```python
from build123d import *

# Parameters (mm, degrees)
SKETCH_1_W               = 50
SKETCH_1_H               = 50
EXTRUDE_1_DEPTH          = 5
CUT_EXTRUDE_1_REACH      = 37.707
SKETCH_2_R               = 15
SKETCH_3_R               = 22.5
CUT_EXTRUDE_2_DEPTH      = 3
CUT_EXTRUDE_3_REACH      = 37.482
SKETCH_4_R               = 1.25
CHAMFER_1_SIZE           = 1
EXTRUDE_2_DEPTH          = 1.5
EXTRUDE_START            = 20
EXTRUDE_3_DEPTH          = 20
CUT_EXTRUDE_4_REACH      = 59.228
SKETCH_9_R               = 1.65
CUT_EXTRUDE_5_DEPTH      = 3
MIRROR_1_COPY_1_REACH    = 59.228
MIRROR_1_COPY_1_SKETCH_R = 1.65
MIRROR_1_COPY_2_DEPTH    = 3


with BuildPart() as part:
    # Sketch 1 → Extrude 1 (new body)
    with BuildSketch(Plane(origin=(0, 0, 0), x_dir=(1, 0, 0), z_dir=(0, 1, 0))):
        Rectangle(SKETCH_1_W, SKETCH_1_H)
    extrude(amount=EXTRUDE_1_DEPTH)

    # Sketch 2 → Cut-Extrude 1 (cut, up to next)
    with BuildSketch(Plane(origin=(0, 5, 0), x_dir=(1, 0, 0), z_dir=(0, 1, 0)), mode=Mode.PRIVATE) as cut_extrude_1_sk1:
        with Locations(Location((0, 0, 0), (0, 0, 270))):
            Circle(SKETCH_2_R)
    cut_extrude_1_tool1 = extrude(cut_extrude_1_sk1.sketch, amount=-CUT_EXTRUDE_1_REACH, mode=Mode.PRIVATE) & part.part
    add(cut_extrude_1_tool1.solids().sort_by_distance((0, 5, 0))[0], mode=Mode.SUBTRACT)

    # Sketch 3 → Cut-Extrude 2 (cut)
    with BuildSketch(Plane(origin=(0, 5, 0), x_dir=(1, 0, 0), z_dir=(0, 1, 0))):
        with Locations(Location((0, 0, 0), (0, 0, 270))):
            Circle(SKETCH_3_R)
    extrude(amount=-CUT_EXTRUDE_2_DEPTH, mode=Mode.SUBTRACT)

    # Sketch 4 → Cut-Extrude 3 (cut, up to next)
    with BuildSketch(Plane(origin=(0, 2, 0), x_dir=(1, 0, 0), z_dir=(0, 1, 0)), mode=Mode.PRIVATE) as cut_extrude_3_sk1:
        with Locations(Location((0, -18.5, 0), (0, 0, 270))):
            Circle(SKETCH_4_R)
    cut_extrude_3_tool1 = extrude(cut_extrude_3_sk1.sketch, amount=-CUT_EXTRUDE_3_REACH, mode=Mode.PRIVATE) & part.part
    # Sketch 4 → Cut-Extrude 3 (cut, up to next)
    with BuildSketch(Plane(origin=(0, 2, 0), x_dir=(1, 0, 0), z_dir=(0, 1, 0)), mode=Mode.PRIVATE) as cut_extrude_3_sk2:
        with Locations(Location((-16.02146997, 9.25, 0), (0, 0, 270))):
            Circle(SKETCH_4_R)
    cut_extrude_3_tool2 = extrude(cut_extrude_3_sk2.sketch, amount=-CUT_EXTRUDE_3_REACH, mode=Mode.PRIVATE) & part.part
    # Sketch 4 → Cut-Extrude 3 (cut, up to next)
    with BuildSketch(Plane(origin=(0, 2, 0), x_dir=(1, 0, 0), z_dir=(0, 1, 0)), mode=Mode.PRIVATE) as cut_extrude_3_sk3:
        with Locations(Location((16.02146997, 9.25, 0), (0, 0, 270))):
            Circle(SKETCH_4_R)
    cut_extrude_3_tool3 = extrude(cut_extrude_3_sk3.sketch, amount=-CUT_EXTRUDE_3_REACH, mode=Mode.PRIVATE) & part.part
    add(cut_extrude_3_tool1.solids().sort_by_distance((0, 2, 18.5))[0], mode=Mode.SUBTRACT)
    add(cut_extrude_3_tool2.solids().sort_by_distance((-16.02147, 2, -9.25))[0], mode=Mode.SUBTRACT)
    add(cut_extrude_3_tool3.solids().sort_by_distance((16.02147, 2, -9.25))[0], mode=Mode.SUBTRACT)

    # Chamfer 1
    chamfer_1_edges = [part.edges().sort_by_distance(p)[0] for p in [
        (0, 2, -22.5),
    ]]
    chamfer(chamfer_1_edges, length=CHAMFER_1_SIZE)

    # Sketch 7 → Extrude 2 (add)
    with BuildSketch(Plane(origin=(0, 2, 0), x_dir=(1, 0, 0), z_dir=(0, 1, 0))):
        with BuildLine():
            ThreePointArc((-5.137558045, 19.173627652), (-9.925, 17.190604265), (-14.036069607, 14.036069607))
            ThreePointArc((-14.036069607, 14.036069607), (-14.036069607, 11.773327907), (-11.773327907, 11.773327907))
            ThreePointArc((-11.773327907, 11.773327907), (-8.325, 14.419322973), (-4.309337101, 16.082665008))
            ThreePointArc((-4.309337101, 16.082665008), (-3.177966251, 18.042256802), (-5.137558045, 19.173627652))
        make_face()
        with BuildLine():
            ThreePointArc((14.036069607, 14.036069607), (9.925, 17.190604265), (5.137558045, 19.173627652))
            ThreePointArc((5.137558045, 19.173627652), (3.177966251, 18.042256802), (4.309337101, 16.082665008))
            ThreePointArc((4.309337101, 16.082665008), (8.325, 14.419322973), (11.773327907, 11.773327907))
            ThreePointArc((11.773327907, 11.773327907), (14.036069607, 11.773327907), (14.036069607, 14.036069607))
        make_face()
        with BuildLine():
            ThreePointArc((19.173627652, -5.137558045), (19.85, 0), (19.173627652, 5.137558045))
            ThreePointArc((19.173627652, 5.137558045), (17.214035858, 6.268928895), (16.082665008, 4.309337101))
            ThreePointArc((16.082665008, 4.309337101), (16.65, 0), (16.082665008, -4.309337101))
            ThreePointArc((16.082665008, -4.309337101), (17.214035858, -6.268928895), (19.173627652, -5.137558045))
        make_face()
        with BuildLine():
            ThreePointArc((5.137558045, -19.173627652), (9.925, -17.190604265), (14.036069607, -14.036069607))
            ThreePointArc((14.036069607, -14.036069607), (14.036069607, -11.773327907), (11.773327907, -11.773327907))
            ThreePointArc((11.773327907, -11.773327907), (8.325, -14.419322973), (4.309337101, -16.082665008))
            ThreePointArc((4.309337101, -16.082665008), (3.177966251, -18.042256802), (5.137558045, -19.173627652))
        make_face()
        with BuildLine():
            ThreePointArc((-14.036069607, -14.036069607), (-9.925, -17.190604265), (-5.137558045, -19.173627652))
            ThreePointArc((-5.137558045, -19.173627652), (-3.177966251, -18.042256802), (-4.309337101, -16.082665008))
            ThreePointArc((-4.309337101, -16.082665008), (-8.325, -14.419322973), (-11.773327907, -11.773327907))
            ThreePointArc((-11.773327907, -11.773327907), (-14.036069607, -11.773327907), (-14.036069607, -14.036069607))
        make_face()
        with BuildLine():
            ThreePointArc((-19.173627652, 5.137558045), (-19.85, 0), (-19.173627652, -5.137558045))
            ThreePointArc((-19.173627652, -5.137558045), (-17.214035858, -6.268928895), (-16.082665008, -4.309337101))
            ThreePointArc((-16.082665008, -4.309337101), (-16.65, 0), (-16.082665008, 4.309337101))
            ThreePointArc((-16.082665008, 4.309337101), (-17.214035858, 6.268928895), (-19.173627652, 5.137558045))
        make_face()
    extrude(amount=EXTRUDE_2_DEPTH)

    # Sketch 8 → Extrude 3 (add)
    with BuildSketch(Plane(origin=(0, 5, 0), x_dir=(1, 0, 0), z_dir=(0, 1, 0)).offset(EXTRUDE_START)):
        with BuildLine():
            Line((-25, -25), (25, -25))
            Line((25, -25), (25, -20))
            Line((25, -20), (10.307764064, -20))
            ThreePointArc((10.307764064, -20), (0, -22.5), (-10.307764064, -20))
            Line((-10.307764064, -20), (-25, -20))
            Line((-25, -20), (-25, -25))
        make_face()
    extrude_3 = extrude(amount=-EXTRUDE_3_DEPTH)

    # Sketch 9 → Cut-Extrude 4 (cut, up to next)
    with BuildSketch(Plane(origin=(0, 0, 20), x_dir=(-1, 0, 0), z_dir=(0, 0, -1)), mode=Mode.PRIVATE) as cut_extrude_4_sk1:
        with Locations((21, 21)):
            Circle(SKETCH_9_R)
    cut_extrude_4_tool1 = extrude(cut_extrude_4_sk1.sketch, amount=-CUT_EXTRUDE_4_REACH, mode=Mode.PRIVATE) & part.part
    # Sketch 9 → Cut-Extrude 4 (cut, up to next)
    with BuildSketch(Plane(origin=(0, 0, 20), x_dir=(-1, 0, 0), z_dir=(0, 0, -1)), mode=Mode.PRIVATE) as cut_extrude_4_sk2:
        with Locations((21, 9)):
            Circle(SKETCH_9_R)
    cut_extrude_4_tool2 = extrude(cut_extrude_4_sk2.sketch, amount=-CUT_EXTRUDE_4_REACH, mode=Mode.PRIVATE) & part.part
    cut_extrude_4_1 = cut_extrude_4_tool1.solids().sort_by_distance((-21, 21, 20))[0]
    add(cut_extrude_4_1, mode=Mode.SUBTRACT)
    cut_extrude_4_2 = cut_extrude_4_tool2.solids().sort_by_distance((-21, 9, 20))[0]
    add(cut_extrude_4_2, mode=Mode.SUBTRACT)
    cut_extrude_4 = cut_extrude_4_1 + cut_extrude_4_2  # Cut-Extrude 4 as one shape, for the pattern or mirror that repeats it

    # Sketch 10 → Cut-Extrude 5 (cut)
    with BuildSketch(Plane(origin=(0, 0, 20), x_dir=(-1, 0, 0), z_dir=(0, 0, -1))):
        Polygon((24.290896534, 21), (22.645448267, 23.85), (19.354551733, 23.85), (17.709103466, 21), (19.354551733, 18.15), (22.645448267, 18.15), align=None)
        Polygon((24.290896534, 9), (22.645448267, 11.85), (19.354551733, 11.85), (17.709103466, 9), (19.354551733, 6.15), (22.645448267, 6.15), align=None)
    cut_extrude_5 = extrude(amount=-CUT_EXTRUDE_5_DEPTH, mode=Mode.SUBTRACT)

    # Mirror 2: Cut-Extrude 4, Cut-Extrude 5 across plane
    add(cut_extrude_4.mirror(Plane(origin=(0, 0, 0), x_dir=(0, 0, 1), z_dir=(1, 0, 0))), mode=Mode.SUBTRACT)
    add(cut_extrude_5.mirror(Plane(origin=(0, 0, 0), x_dir=(0, 0, 1), z_dir=(1, 0, 0))), mode=Mode.SUBTRACT)

    # Mirror 1: Extrude 3, Cut-Extrude 4, Cut-Extrude 5 across plane
    add(extrude_3.mirror(Plane.XY))
    add(cut_extrude_4.mirror(Plane.XY), mode=Mode.SUBTRACT)
    add(cut_extrude_5.mirror(Plane.XY), mode=Mode.SUBTRACT)

    # Mirror 1 copy 1 sketch → Mirror 1 copy 1 (cut, up to next)
    with BuildSketch(Plane.XY.offset(-20), mode=Mode.PRIVATE) as mirror_1_copy_1_sk1:
        with Locations((21, 21)):
            Circle(MIRROR_1_COPY_1_SKETCH_R)
    mirror_1_copy_1_tool1 = extrude(mirror_1_copy_1_sk1.sketch, amount=-MIRROR_1_COPY_1_REACH, mode=Mode.PRIVATE) & part.part
    # Mirror 1 copy 1 sketch → Mirror 1 copy 1 (cut, up to next)
    with BuildSketch(Plane.XY.offset(-20), mode=Mode.PRIVATE) as mirror_1_copy_1_sk2:
        with Locations((21, 9)):
            Circle(MIRROR_1_COPY_1_SKETCH_R)
    mirror_1_copy_1_tool2 = extrude(mirror_1_copy_1_sk2.sketch, amount=-MIRROR_1_COPY_1_REACH, mode=Mode.PRIVATE) & part.part
    add(mirror_1_copy_1_tool1.solids().sort_by_distance((21, 21, -20))[0], mode=Mode.SUBTRACT)
    add(mirror_1_copy_1_tool2.solids().sort_by_distance((21, 9, -20))[0], mode=Mode.SUBTRACT)

    # Mirror 1 copy 2 sketch → Mirror 1 copy 2 (cut)
    with BuildSketch(Plane.XY.offset(-20)):
        Polygon((24.290896534, 21), (22.645448267, 23.85), (19.354551733, 23.85), (17.709103466, 21), (19.354551733, 18.15), (22.645448267, 18.15), align=None)
        Polygon((24.290896534, 9), (22.645448267, 11.85), (19.354551733, 11.85), (17.709103466, 9), (19.354551733, 6.15), (22.645448267, 6.15), align=None)
    extrude(amount=-MIRROR_1_COPY_2_DEPTH, mode=Mode.SUBTRACT)


solid = part.part
```
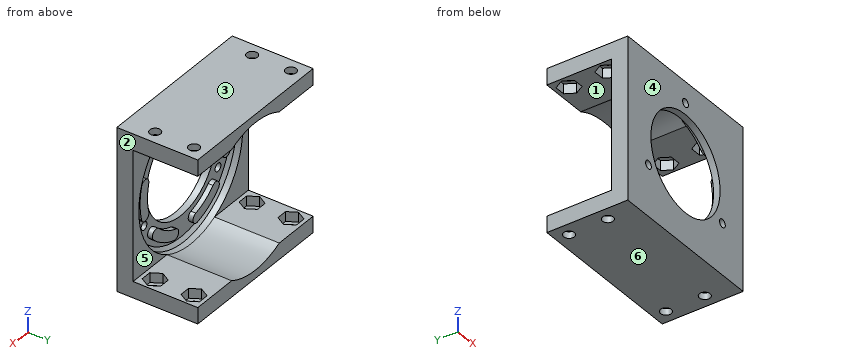
The model under review builds one solid part; all positions refer to its coordinate system, in mm. Face numbers are marked on the shaded views. A direction names the side the tool comes from. Round coordinates to 2 decimals unless told otherwise and drop trailing zeros. Loops run counter-clockwise (first coordinate to the right, second up) from the corner with the lowest first, then second, coordinate; pieces in that order, holes last. Notation, with made-up numbers: (83, 59.5) - (104, 59.5) arc R12 ccw to (104, 68.5) - close; hole circle Ø10 at (73, -29.5). An arc over 180 degrees is marked (long way). Write each question's results on one line, items separated by ' | '. Start each with the question number.
Q1. Draft analysis for pull direction Z (two halves, no side actions). For the marked faces 3, 4, 5 and 6, state which applies: pulls with the +Z half, pulls with the -Z half, needs draft (parallel to the pull), parting line crosses it, or undercut.
Q2. Take a section at A-A on x = 0. Give the boundary of the cut face in (y, z), plus the area to 3 significant figures.
Q3. Wall thickness on line 1 along Y through (x, z) = (-21, 24); line 2 along X through (y, z) = (0.75, 18.5); line 3 along X through (y, z) = (2.25, -14): over which ranges is each line inside the solid? List them lowest first. Write a range as [from, to].
Q4. Tool access review of the marked faces 1 and 2: name each direction out of +Z, -Z, +X, -X, +Y, -Y from which nothing blocks a thin tool from reaching the whole face with its end or side.
Q5. Insertion check: P1, Ø3, axis at x = -12.5, z = -15.5, coming from the +Y side; P2, Ø4.5, axis at x = -21, y = 9, coming from the -Z side; P3, Ø2, axis at x = 15, z = -2, coming from the +Y side; P4, Ø24, axis at x = 0, z = 0, coming from the -Y side. Each pin has a flat end and moves straight along its axis. Give the tip position at first contact, or say it passes through.
Q6. Take a section at B-B on z = -9.25. Give the number of separate pieces and of enclosed holes in the cut face, plus the area to 3 significant figures.
Data:
1) face 3: pulls with the +Z half | face 4: needs draft | face 5: undercut | face 6: pulls with the -Z half
2) outline: (0, -25) - (25, -25) - (25, -22.5) - (3, -22.5) - (2, -21.5) - (2, -15) - (0, -15) - close; (0, 15) - (2, 15) - (2, 17.25) - (0, 17.25) - close; (0, 19.75) - (2, 19.75) - (2, 21.5) - (3, 22.5) - (25, 22.5) - (25, 25) - (0, 25) - close | area: 151 mm²
3) line 1: y = [0, 7.35], [10.65, 19.35], [22.65, 25] | line 2: x = [-25, -1.25], [1.25, 25] | line 3: x = [-25, -16.65], [-14.07, -9.01], [9.01, 14.07], [16.65, 25]
4) face 1: +X, -X, +Y | face 2: +Z, -Z, +X, +Y, -Y
5) P1: stops at y = 3.5 | P2: stops at z = -25 | P3: stops at y = 2 | P4: passes through
6) separate pieces: 4 | enclosed holes: 0 | area: 70.8 mm²
